Study the drawing (mm; zero at the part's minimum x, y, z) and answer. Round coordinates to 2 decimals unless told otherwise and drop trailing zeros. Write each loop counter-clockwise with the first axis right and the second up, starting at its lowest first coordinate (ties: lowest second). Pieces come first, ordered by that corner, then holes.
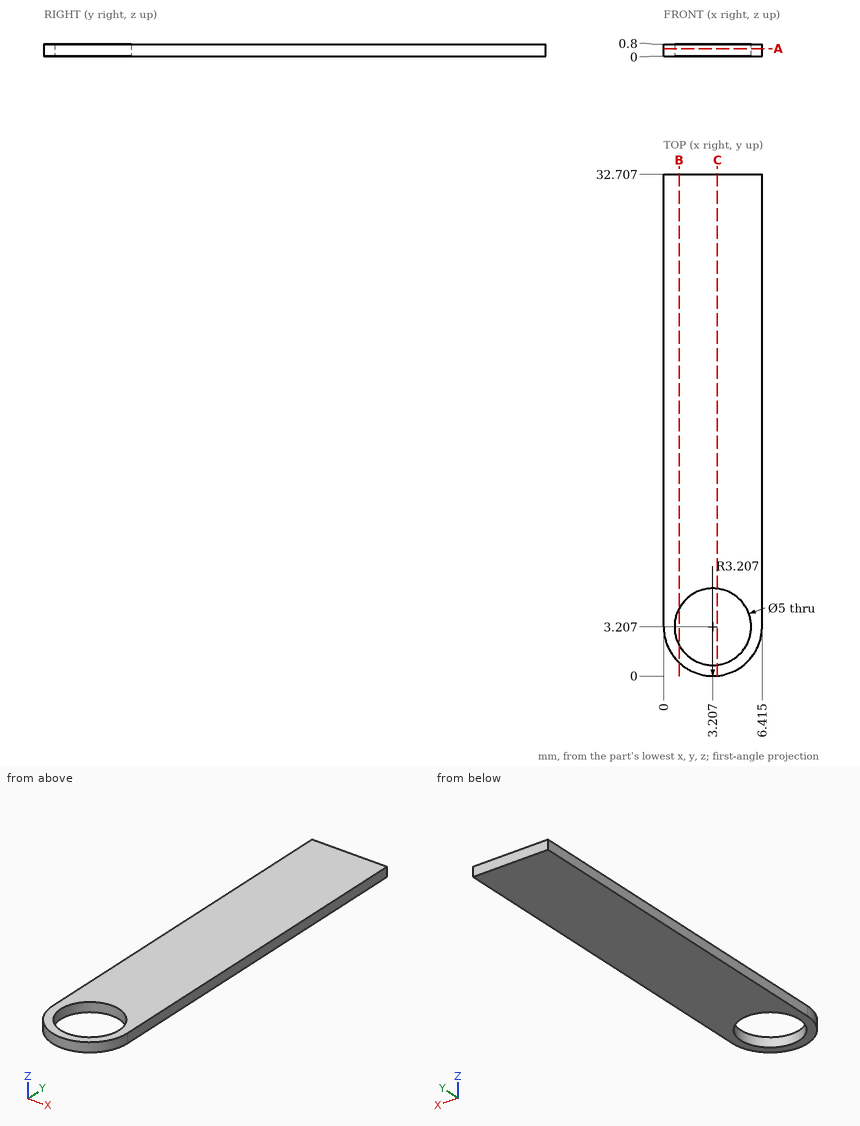
1. Straight lines are drawn through the part: line 1 along X through (y, z) = (2, 0.7) (1 decimal); line 2 along Y through (x, z) = (1.5, 0.1) (1 decimal); line 3 along Y through (x, z) = (2, 0.25) (1 decimal). For each, find the intervals that lie inside material, in ascending order.
Geometry says:
line 1: x = 0.2 to 1, 5.4 to 6.2
line 2: y = 0.5 to 1.4, 5 to 32.7
line 3: y = 0.2 to 1, 5.4 to 32.7
2. Section A-A on z = 0.5 is taken. Determine the outline of the cut face in (x, y) (1 decimal).
Geometry says:
outline: (0, 3.2) arc R3.2 ccw to (6.4, 3.2) - (6.4, 32.7) - (0, 32.7) - close; hole circle Ø5 at (3.2, 3.2)
3. Section C-C on x = 3.5 is taken. Determine the outline of the cut face in (y, z) (1 decimal).
Geometry says:
outline: (0, 0) - (0.7, 0) - (0.7, 0.8) - (0, 0.8) - close; (5.7, 0) - (32.7, 0) - (32.7, 0.8) - (5.7, 0.8) - close
4. Section B-B on x = 1 is taken. Determine the outline of the cut face in (y, z).
Geometry says:
outline: (0.88, 0) - (2.03, 0) - (2.03, 0.8) - (0.88, 0.8) - close; (4.38, 0) - (32.71, 0) - (32.71, 0.8) - (4.38, 0.8) - close
